Read the model definition and answer for the solid it produces. Units are mm, in the model's axes. Face numbers are marked on the shaded views. A direction names the side the tool comes from. Coordinates: 2 decimals unless noted, no trailing zeros. Write each loop counter-clockwise with the first axis right and the second up, starting at its lowest first coordinate (ties: lowest second). Pieces come first, ordered by that corner, then holes.
(1) Which of the six approach directions +Z, -Z, +X, -X, +Y, -Y give full straight-line access (tool end or side, diameter ignored) to the marked faces 5, 6, 7 and 8?
(2) Given pin 1 (3 mm diameter, centred on y = 2, z = 17.5, fed in from -X); pin 2 (12 mm diameter, centred on x = 2.5, z = 22, fed in from -Y); pin 3 (1 mm diameter, centred on y = 3.5, z = 14.5, fed in from +X), each flat-ended and moving along its own axis, determine where each tip first touches the part or whether it passes through.
(3) Section A-A on z = 14.5 is taken. Write down the section's boundary in (x, y), then the cut area to 3 significant figures.
(4) Find the intervals of material crossed by probe 1 along X at (y, z) = (0.25, 15.75); probe 2 along Y at (x, z) = (0, 14); probe 3 along Y at (x, z) = (6, 12), in increasing order.
(5) The mould has two halves that part along Y. Classify the marked faces 1, 2, 3 and 4: +Y half, -Y half, draft (parallel to the pull), parting line (faces both ways), or undercut.
(6) Section B-B on x = 0 is taken. Write down the section's boundary in (y, z) (3 decimals), then the cut area to 3 significant figures.
(7) Section D-D on z = 9 is taken. Write down the section's boundary in (x, y), then the cut area to 3 significant figures.
from build123d import *

# Parameters (mm, degrees)
F0_W     = 20.03
F0_H     = 20.03
F1_DEPTH = 5
F2_W     = 15.6
F2_H     = 15.6
F3_DEPTH = 20
F4_R     = 5.5
F5_DEPTH = 15
F6_R     = 1


with BuildPart() as f1:
    # F0 (on Top) → F1 (new body)
    with BuildSketch(Plane.XY):
        Rectangle(F0_W, F0_H)
    extrude(amount=F1_DEPTH)

    # F2 (on face) → F3 (join)
    with BuildSketch(Plane.XY.offset(5)):
        Rectangle(F2_W, F2_H)
    extrude(amount=F3_DEPTH)

    # F4 (on face) → F5 (cut)
    with BuildSketch(Plane.XY.offset(25)):
        Circle(F4_R)
    extrude(amount=-F5_DEPTH, mode=Mode.SUBTRACT)

    # F6
    f6_edges = [f1.edges().sort_by_distance(p)[0] for p in [
        (-7.8, -7.8, 15),
        (7.8, -7.8, 15),
        (7.8, 7.8, 15),
        (-7.8, 7.8, 15),
    ]]
    fillet(f6_edges, radius=F6_R)


solid = f1.part
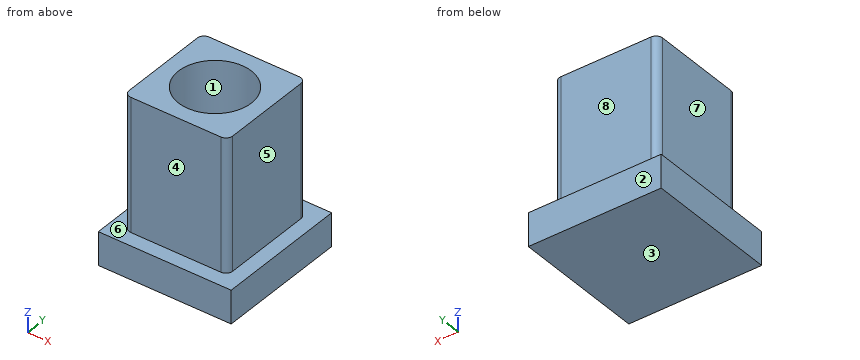
Response:
1. face 5: +Z, +X, +Y, -Y
1. face 6: +Z
1. face 7: +Z, -X, +Y, -Y
1. face 8: +Z, +X, -X, +Y
2. pin 1: stops at x = -7.8
2. pin 2: stops at y = -7.8
2. pin 3: stops at x = 7.8
3. outline: (-7.8, -6.8) arc R1 ccw to (-6.8, -7.8) - (6.8, -7.8) arc R1 ccw to (7.8, -6.8) - (7.8, 6.8) arc R1 ccw to (6.8, 7.8) - (-6.8, 7.8) arc R1 ccw to (-7.8, 6.8) - close; hole circle Ø11 at (0, 0)
3. area: 147 mm2
4. probe 1: x = -7.8 to -5.49, 5.49 to 7.8
4. probe 2: y = -7.8 to -5.5, 5.5 to 7.8
4. probe 3: y = -7.8 to 7.8
5. face 1: undercut
5. face 2: +Y half
5. face 3: draft
5. face 4: -Y half
6. outline: (-10.015, 0) - (10.015, 0) - (10.015, 5) - (7.8, 5) - (7.8, 25) - (5.5, 25) - (5.5, 10) - (-5.5, 10) - (-5.5, 25) - (-7.8, 25) - (-7.8, 5) - (-10.015, 5) - close
6. area: 247 mm2
7. outline: (-7.8, -6.8) arc R1 ccw to (-6.8, -7.8) - (6.8, -7.8) arc R1 ccw to (7.8, -6.8) - (7.8, 6.8) arc R1 ccw to (6.8, 7.8) - (-6.8, 7.8) arc R1 ccw to (-7.8, 6.8) - close
7. area: 243 mm2
